Autodesk Inventor part; units mm, degrees
ref_plane "Piano iniziale" through (0, 0, 0) normal (0, 0, 1) x (1, 0, 0)
ref_plane "Piano finale" through (0, 0, 200) normal (0, 0, 1) x (1, 0, 0)
ref_plane "YZ Plane" through (0, 0, 0) normal (1, 0, 0) x (0, 1, 0)
ref_plane "Piano iniziale" through (0, 0, 0) normal (0, 0, 1) x (1, 0, 0)
ref_plane "Piano finale" through (0, 0, 200) normal (0, 0, 1) x (1, 0, 0)
sketch "Schizzo" plane through (0, 0, 0) normal (0, 0, 1) x (1, 0, 0)
  line L0 (-10, -6) -> (-10, 6)
  line L1 (-6, 10) -> (6, 10)
  line L2 (10, 6) -> (10, -6)
  line L3 (6, -10) -> (-6, -10)
  arc A0 (-10, -6) -> (-6, -10) centre (-6, -6) ccw
  arc A1 (10, 6) -> (6, 10) centre (6, 6) ccw
  arc A2 (-6, 10) -> (-10, 6) centre (-6, 6) ccw
  arc A3 (6, -10) -> (10, -6) centre (6, -6) ccw
  arc A4 (-6, 8) -> (-8, 6) centre (-6, 6) ccw
  line L4 (-6, 8) -> (6, 8)
  arc A5 (8, 6) -> (6, 8) centre (6, 6) ccw
  line L5 (8, 6) -> (8, -6)
  arc A6 (6, -8) -> (8, -6) centre (6, -6) ccw
  line L6 (6, -8) -> (-6, -8)
  arc A7 (-8, -6) -> (-6, -8) centre (-6, -6) ccw
  line L7 (-8, -6) -> (-8, 6)
  line L8 (0, 15.1598) -> (0, -15.1598) construction
  line L9 (-15.1598, 0) -> (15.1598, 0) construction
  dimension "d7" = 4
  dimension "d9" = 20
  dimension "d11" = 20
  dimension "d12" = 2
  dimension "d15" = 10
  dimension "d16" = 10
extrude "Corpo" add sketch "Schizzo" along normal up to surface (200 mm away) from surface at 0
sketch "Sketch3" plane through (0, 0, 0) normal (0, 0, 1) x (1, 0, 0)
  line L0 (0, 0) -> (10, 0)
ref_plane "Work Plane3" through (0, 0, 0) normal (0, -1, 0) x (1, 0, 0)
sketch "Sketch4" plane through (0, 0, 0) normal (0, -1, 0) x (1, 0, 0)
  line L0 (-2, 0) -> (12, 0)
  line L1 (-2, 200) -> (12, 200)
  dimension "d18" = 200
sketch "Schizzo5" plane through (-6, -10, 0) normal (0, -1, 0) x (1, 0, 0)
  line L0 (-4, 0) -> (0, 0)
  line L1 (-4, 0) -> (27.2685, 31.2685)
  line L2 (-4, 0) -> (40.2203, 0) construction
  line L3 (27.2685, 31.2685) -> (27.2685, 0)
  line L4 (27.2685, 0) -> (-4, 0)
  line L5 (-4, 200) -> (31.4981, 164.5019)
  line L6 (-4, 200) -> (46.2019, 200) construction
  line L7 (31.4981, 164.5019) -> (31.4981, 200)
  line L8 (31.4981, 200) -> (-4, 200)
  point P0 (6, 0)
  dimension "d19" = 45
  dimension "d20" = 45
extrude "Estrusione2" cut sketch "Schizzo5" against normal up to next
sketch "Schizzo6" plane through (-10, 6, 0) normal (-1, 0, 0) x (0, 0, 1)
  line L0 (0, -12) -> (0, 0)
  line L1 (200, -12) -> (200, 0)
  point P0 (0, -6)
  point P1 (190, -6)
  point P2 (0, -6)
  dimension "d23" = 10
hole "Foro1" at (-10, 0, 190) direction (1, 0, 0) diameter 10 end through all
equation "\"d7\" = G_IR"
equation "\"d9\" = G_W"
equation "\"d11\" = G_H"
equation "\"d12\" = G_T"
equation "\"d15\" = 0.5 * d9"
equation "\"d16\" = 0.5 * d11"
equation "\"d3\" = G_L"
equation "\"G_W\" = 20"
equation "\"G_H\" = 20"
equation "\"G_T\" = 2"
equation "\"G_IR\" = 4"
equation "\"G_L\" = d18"
equation "\"G_OFFSET_START\" = 0"
equation "\"G_OFFSET_END\" = 0"
properties part number "ISO 10799-2 - 20x20x2 - 200" material "Acciaio, Dolce"
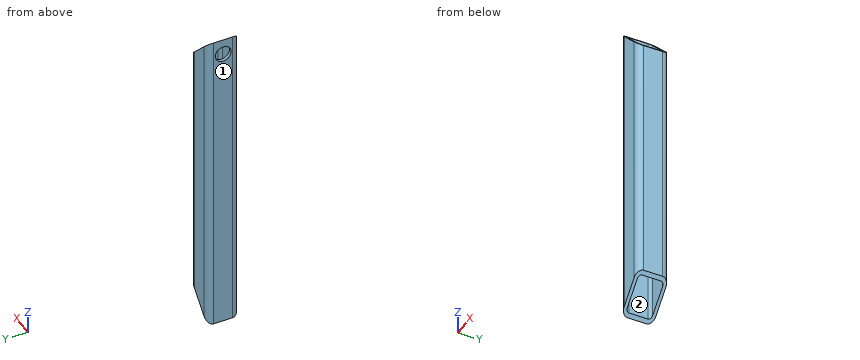
Input: part model. Units: mm. Frame: model coordinates. Face numbers are marked on the shaded views. A direction names the side the tool comes from. Round coordinates to 2 decimals unless told otherwise and drop trailing zeros. Order: outer loops, then holes, each group sorted by start corner. A loop starts at its lowest first (then second) coordinate and runs counter-clockwise, first axis right, second up. Notation, with made-up numbers: (-4, 79) - (44, 79) arc R9 ccw to (44, 87) - close; hole circle Ø10 at (-33.5, 45). An arc over 180 degrees is marked (long way). Use a Markdown table: item, result.
1. Section B-B on y = 0. Return the cut outline in (x, z), then the cut area to 3 significant figures.
Evaluation:
| item | result |
|---|---|
| outline | (-10, 0) - (-8, 2) - (-8, 185) - (-10, 185) - close; (-10, 195) - (-8, 195) - (-8, 198) - (-10, 200) - close; (8, 18) - (10, 20) - (10, 180) - (8, 182) - close |
| area | 700 mm^2 |
2. Section C-C on z = 99.5. Return the cut outline in (x, y).
Evaluation:
| item | result |
|---|---|
| outline | (-10, -6) arc R4 ccw to (-6, -10) - (6, -10) arc R4 ccw to (10, -6) - (10, 6) arc R4 ccw to (6, 10) - (-6, 10) arc R4 ccw to (-10, 6) - close; hole (-8, -6) arc R2 ccw to (-6, -8) - (6, -8) arc R2 ccw to (8, -6) - (8, 6) arc R2 ccw to (6, 8) - (-6, 8) arc R2 ccw to (-8, 6) - close |
3. Section D-D on z = 190. Return the cut outline in (x, y).
Evaluation:
| item | result |
|---|---|
| outline | (-10, -6) arc R4 ccw to (-6, -10) - (0, -10) - (0, -8) - (-6, -8) arc R2 cw to (-8, -6) - (-8, -5) - (-10, -5) - close; (-10, 5) - (-8, 5) - (-8, 6) arc R2 cw to (-6, 8) - (0, 8) - (0, 10) - (-6, 10) arc R4 ccw to (-10, 6) - close |
4. Access query for the marked faces 1 and 2. Directions: +Z, -Z, +X, -X, +Y, -Y. A direction counts if a zero-diameter tool reaches every point of the face in a straight line with its end or side. Return the directions, or none.
Evaluation:
| item | result |
|---|---|
| face 1 | +Z, -Z, -X, +Y, -Y |
| face 2 | +Z, -Z |
5. Section A-A on x = 0.5. Return the cut outline in (y, z).
Evaluation:
| item | result |
|---|---|
| outline | (-10, 10.5) - (-8, 10.5) - (-8, 189.5) - (-10, 189.5) - close; (8, 10.5) - (10, 10.5) - (10, 189.5) - (8, 189.5) - close |
6. Material intervals for probe 1 along X at (y, z) = (-5.25, 73); probe 2 along Y at (x, z) = (-9, 190), sorted ascending.
Evaluation:
| item | result |
|---|---|
| probe 1 | -10 to -8, 8 to 10 |
| probe 2 | -8.65 to -5, 5 to 8.65 |
